Verification items for the finished model (mm, model axes). Face numbers are marked on the shaded views. A direction names the side the tool comes from. Give positions to 0.01 mm unless a question says otherwise; leave off trailing zeros. Order: outer loops, then holes, each group sorted by start corner. A loop starts at its lowest first (then second) coordinate and runs counter-clockwise, first axis right, second up.
Autodesk Inventor part; units mm, degrees
ref_plane "Work Plane2" through (0, 0, 0) normal (1, 0, 0) x (0, 0, -1)
ref_plane "YZ Plane" through (0, 0, 0) normal (1, 0, 0) x (0, 1, 0)
ref_plane "XZ Plane" through (0, 0, 0) normal (0, 1, 0) x (-1, 0, 0)
sketch "Sketch1" plane through (0, 0, 0) normal (0, 0, 1) x (1, 0, 0)
  circle A0 centre (0, 0) radius 12.7
  circle A1 centre (0, 0) radius 16.7005
  dimension "d0" = 25.4
  dimension "d1" = 33.401
extrude "Extrusion1" add sketch "Sketch1" against normal blind 53.975 contours A0
ref_plane "Work Plane1" through (0, 0, -25.4) normal (0, 0, 1) x (1, 0, 0)
sketch "Sketch3" plane through (0, 0, -25.4) normal (0, 0, 1) x (1, 0, 0)
  circle A0 centre (0, 0) radius 16.7005
  dimension "d6" = 33.401
extrude "Extrusion2" add sketch "Sketch3" against normal blind 3.175
sketch "Sketch4" plane through (0, 0, -53.975) normal (0, 0, -1) x (-1, 0, 0)
  line L0 (0, 0) -> (0, 16.7005)
  circle A0 centre (0, 0) radius 16.7005
ref_plane "Work Plane2" through (0, 0, 0) normal (1, 0, 0) x (0, 0, -1)
sketch "Sketch5" plane through (0, 0, 0) normal (1, 0, 0) x (0, 0, -1)
  line L0 (53.975, -12.7) -> (53.975, 12.7)
  circle A0 centre (53.975, 0) radius 19.05
  point P0 (0, 0)
  dimension "d9" = 38.1
extrude "Extrusion3" cut sketch "Sketch5" along normal blind 12.7
extrude "Extrusion4" add sketch "Sketch5" against normal blind 20.32
properties part number "Adjustable elbow piece 1 inch"
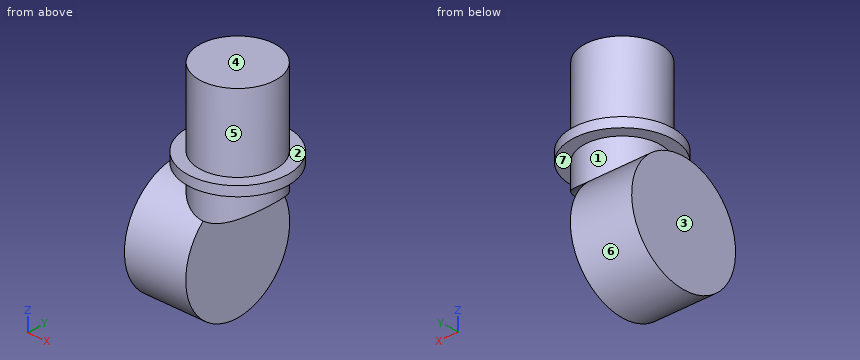
(1) Section check B-B, the plane y = 0. Enter the section's corners in (x, z) (1 decimal), then the cut area to 3 significant figures.
Solved:
outline: (-20.3, -73) - (0, -73) - (0, -34.9) - (12.7, -34.9) - (12.7, -28.6) - (16.7, -28.6) - (16.7, -25.4) - (12.7, -25.4) - (12.7, 0) - (-12.7, 0) - (-12.7, -25.4) - (-16.7, -25.4) - (-16.7, -28.6) - (-12.7, -28.6) - (-12.7, -34.9) - (-20.3, -34.9) - close
area: 1,690 mm2
(2) Release check for a two-part mould opening along Z. For the marked faces 1, 2 and 3 record: pulls with the +Z half, pulls with the -Z half, needs draft (parallel to the pull), parting line crosses it, or undercut.
Solved:
face 1: undercut
face 2: pulls with the +Z half
face 3: needs draft
(3) Section check C-C, the plane x = -14.5. Enter the section's corners in (y, z) (3 decimals), then the cut area to 3 significant figures.
Solved:
outline: circle Ø38.1 at (0, -53.975); (-8.286, -28.575) - (8.286, -28.575) - (8.286, -25.4) - (-8.286, -25.4) - close
area: 1,190 mm2
(4) Set-up check for the marked faces 4, 5, 6 and 7: record each of +Z, -Z, +X, -X, +Y, -Y from which the full face is reachable in a straight line by a thin tool's end or side.
Solved:
face 4: +Z, +X, -X, +Y, -Y
face 5: +Z
face 6: -X
face 7: none
(5) Scan lines: line 1 (X direction, y = 16, z = -57.5); line 2 (Z direction, x = -10, y = -8.5) (3 decimals); line 3 (Z direction, x = 15, y = 6.5) (3 decimals). Record each from-to range of solid material in increasing order.
Solved:
line 1: x = -20.32 to 0
line 2: z = -71.024 to -36.926, -28.575 to -25.4
line 3: z = -28.575 to -25.4
(6) Section check A-A, the plane y = 15. Enter the section's corners in (x, z) (3 decimals), then the cut area to 3 significant figures.
Solved:
outline: (-20.32, -65.718) - (0, -65.718) - (0, -42.232) - (-20.32, -42.232) - close; (-7.342, -28.575) - (7.342, -28.575) - (7.342, -25.4) - (-7.342, -25.4) - close
area: 524 mm2
(7) Section check D-D, the plane z = -34. Enter the section's corners in (x, y).
Solved:
outline: circle Ø25.4 at (0, 0)
(8) Go/stop test with flat-tipped pins: pin 1 (10 mm diameter, centred on x = -9.5, y = 13.5, fed in from -Z); pin 2 (2 mm diameter, centred on x = -2.5, y = -11, fed in from -Z); pin 3 (6 mm diameter, centred on x = 9.5, y = -13.5, fed in from -Z) (3 decimals). Record where each tip stops, or that it passes through.
Solved:
pin 1: stops at z = -71.02
pin 2: stops at z = -70.19
pin 3: stops at z = -28.575
